Read the model definition and answer for the solid it produces. Units are mm, in the model's axes. Give positions to 0.01 mm unless a question says otherwise; leave off trailing zeros. Order: outer loops, then holes, each group sorted by start corner. A loop starts at its lowest first (then second) coordinate and runs counter-clockwise, first axis right, second up. Notation, with made-up numbers: (61, 87.25) - (106, 87.25) arc R31 cw to (106, 111.25) - close; hole circle Ø8 at (43.5, 0.25). An arc over 180 degrees is marked (long way). Write item = value, one per line.
Autodesk Inventor part; units mm, degrees
ref_plane "XZ Plane" through (0, 0, 0) normal (0, 1, 0) x (-1, 0, 0)
ref_plane "XY Plane" through (0, 0, 0) normal (0, 0, 1) x (1, 0, 0)
sketch "Sketch1" plane through (0, 0, 0) normal (0, 0, 1) x (1, 0, 0)
  circle A0 centre (0, 0) radius 53.34
  dimension "d0" = 106.68
extrude "Extrusion1" add sketch "Sketch1" along normal mid plane 6.35
sketch "Sketch2" plane through (0, 0, -3.175) normal (0, 0, -1) x (-1, 0, 0)
  point P0 (0, 0)
sketch "Sketch3" plane through (0, 0, -3.175) normal (0, 0, -1) x (-1, 0, 0)
  line L0 (29.9214, 21.4747) -> (33.5583, -15.1753)
  line L1 (33.5583, -15.1753) -> (3.6369, -36.65)
  line L2 (3.6369, -36.65) -> (-29.9214, -21.4747)
  line L3 (-29.9214, -21.4747) -> (-33.5583, 15.1753)
  line L4 (-33.5583, 15.1753) -> (-3.6369, 36.65)
  line L5 (-3.6369, 36.65) -> (29.9214, 21.4747)
  point P0 (0, 0)
  point P1 (0, 0)
  dimension "d3" = 36.83
hole "Hole1" at (33.5583, 15.1753, -3.175) at (3.6369, 36.65, -3.175) at (-29.9214, 21.4747, -3.175) at (-33.5583, -15.1753, -3.175) at (-3.6369, -36.65, -3.175) at (29.9214, -21.4747, -3.175) direction (0, 0, 1) diameter 25.6794 end through all
sketch "Sketch4" plane through (0, 0, -3.175) normal (0, 0, -1) x (-1, 0, 0)
  circle A0 centre (0, 0) radius 6.35
  dimension "d11" = 12.7
extrude "Extrusion2" add sketch "Sketch4" along normal blind 9.525
sketch "Sketch5" plane through (0, 0, -12.7) normal (0, 0, -1) x (-1, 0, 0)
  circle A0 centre (0, 0) radius 6.35
hole "Hole2" at (0, 0, -12.7) direction (0, 0, 1) diameter 5.08 end through all
ref_plane "Work Plane1" through (6.35, 0, 0) normal (1, 0, 0) x (0, 1, 0)
sketch "Sketch6" plane through (6.35, 0, 0) normal (1, 0, 0) x (0, 1, 0)
  line L0 (-6.35, -12.7) -> (6.35, -12.7)
  point P0 (0, 0)
  point P1 (0, -9.525)
  dimension "d22" = 3.175
hole "Hole3" at (6.35, 0, -9.525) direction (-1, 0, 0) diameter 2.159 depth 6.35 tip angle 118
sketch "Sketch7" plane through (0, 0, 3.175) normal (0, 0, 1) x (1, 0, 0)
  circle A0 centre (0, 0) radius 2.54
  line L0 (0, 0) -> (-21.9781, 48.6017)
  circle A1 centre (0, 0) radius 53.34
  circle A2 centre (-29.9214, 21.4747) radius 12.8397
  line L1 (-29.9214, 21.4747) -> (3.4827, 36.5803)
  line L2 (3.4827, 36.5803) -> (3.4827, 23.8112)
  circle A3 centre (3.6369, 36.65) radius 12.8397
  line L3 (3.4827, 36.5803) -> (-8.5593, 40.6638)
  line L4 (-21.9781, 48.6017) -> (-19.3657, 42.8249)
  dimension "d30" = 12.7155
  dimension "d31" = 5.5753
hole "Hole4" at (-19.3657, 42.8249, 3.175) direction (0, 0, -1) diameter 2.6416 end through all
properties part number "threaded filter wheel"
1. Section A-A (y = 32) is taken. Determine the outline of the cut face in (x, z) (3 decimals), and give its area (3 significant figures).
Recorded:
outline = (-42.675, -3.175) - (-37.275, -3.175) - (-37.275, 3.175) - (-42.675, 3.175) - close; (-22.568, -3.175) - (-8.331, -3.175) - (-8.331, 3.175) - (-22.568, 3.175) - close; (15.605, -3.175) - (42.675, -3.175) - (42.675, 3.175) - (15.605, 3.175) - close
area = 297 mm^2
2. Section D-D (x = 0) is taken. Determine the outline of the cut face in (y, z) (3 decimals).
Recorded:
outline = (-53.34, -3.175) - (-48.964, -3.175) - (-48.964, 3.175) - (-53.34, 3.175) - close; (-24.336, -3.175) - (-6.35, -3.175) - (-6.35, -12.7) - (-2.54, -12.7) - (-2.54, 3.175) - (-24.336, 3.175) - close; (2.54, -12.7) - (6.35, -12.7) - (6.35, -3.175) - (24.336, -3.175) - (24.336, 3.175) - (2.54, 3.175) - close; (48.964, -3.175) - (53.34, -3.175) - (53.34, 3.175) - (48.964, 3.175) - close
3. Flat-ended cylindrical pins translate along their axes: pin 1 (20.5 mm diameter, centred on x = -3.64, y = -36.65, fed in from -Z); pin 2 (8 mm diameter, centred on x = -28, z = -0.5, fed in from -Y); pin 3 (3 mm diameter, centred on y = 0, z = -9.525, fed in from +X); pin 4 (8 mm diameter, centred on y = -6.5, z = 0.5, fed in from -X). Find the tip coordinate at first contact, or state that the pin passes through.
Recorded:
pin_1 = through
pin_2 = -47.64
pin_3 = 6.35
pin_4 = -53.28
4. Straight lines are drawn through the part: L1, parallel to Y at x = -32.5, z = -2.5; L2, parallel to Y at x = 32, z = -0.75 (3 decimals); L3, parallel to X at y = -42, z = 0. For each, find the intervals that lie inside material, in ascending order. Write a range as [from, to].
Recorded:
L1 = [-42.3, -27.97], [-2.38, 8.9], [34.05, 42.3]
L2 = [-42.675, -34.145], [-8.804, 2.431], [27.92, 42.675]
L3 = [-32.88, -15.31], [8.04, 32.88]
5. Section C-C (z = 1) is taken. Count the separate pieces of the cut face and the enclosed holes in it, and give its area (3 significant figures).
Recorded:
separate_pieces = 1
enclosed_holes = 8
area = 5,810 mm^2
6. Section B-B (x = 15) is taken. Determine the outline of the cut face in (y, z) (3 decimals).
Recorded:
outline = (-51.187, -3.175) - (30.672, -3.175) - (30.672, 3.175) - (-51.187, 3.175) - close; (42.628, -3.175) - (51.187, -3.175) - (51.187, 3.175) - (42.628, 3.175) - close
7. Determine the mould class of faces 1 (the face through (-34.123, -28.003, 0.044)), 2 (the face through (-6.057, -1.907, -7.871)), 3 (the face through (11, 1, 3.175)) for opening direction Y: +Y half, -Y half, draft (parallel to the pull), parting line (faces both ways), or undercut.
Recorded:
face_1 = undercut
face_2 = parting line
face_3 = draft
